from build123d import *

# Parameters (mm, degrees)
CUT_EXTRUDE_1_DEPTH = 3
FILLET_1_R          = 1
CHAMFER_1_SIZE      = 0.5


with BuildPart() as part:
    # 草图1 → 旋转1 (revolve)
    with BuildSketch(Plane.XY):
        Polygon((0, 0), (0, 5), (4.5, 5), (4.5, 3), (20.5, 3), (20.5, 2.5), (30.5, 2.5), (30.5, 0), align=None)
    revolve(axis=Axis((0, 0, 0), (1, 0, 0)))

    # 草图2 → 切除-拉伸1 (cut)
    with BuildSketch(Plane.ZY):
        Polygon((0, 1.732050808), (-1.5, 0.866025404), (-1.5, -0.866025404), (0, -1.732050808), (1.5, -0.866025404), (1.5, 0.866025404), align=None)
    extrude(amount=-CUT_EXTRUDE_1_DEPTH, mode=Mode.SUBTRACT)

    # 圆角1
    fillet_1_edges = [part.edges().sort_by_distance(p)[0] for p in [
        (0, -5, 0),
    ]]
    fillet(fillet_1_edges, radius=FILLET_1_R)

    # 倒角1
    chamfer_1_edges = [part.edges().sort_by_distance(p)[0] for p in [
        (30.5, -2.5, 0),
    ]]
    chamfer(chamfer_1_edges, length=CHAMFER_1_SIZE)


solid = part.part
CAD build for the part. Positions are in the model's coordinates, mm. A direction names the side the tool comes from. Give positions to 0.01 mm unless a question says otherwise; leave off trailing zeros. Loops run counter-clockwise (first coordinate to the right, second up) from the corner with the lowest first, then second, coordinate; pieces in that order, holes last. Notation, with made-up numbers: M -32,33.25 L 10,33.25 A7 ccw 10,44.25 Z; hole C 80.25,17.5 d1. An arc over 180 degrees is marked long. Answer in a Markdown table with one row per item. Add a question column.
Item 1: Tool access for faces 1 (the face through (13, -3, 0)), 2 (the face through (0, -2, 0)), 3 (the face through (3, 0, 0)): list every direction of +Z, -Z, +X, -X, +Y, -Y with a clear straight run to the whole face (end or side of a thin tool).
Item 2: Band-saw the part on C-C on x = 22. Give the cut face in (y, z).
Item 3: Probe probe 1 along Z at (x, y) = (29, -2); probe 2 along X at (y, z) = (-1.5, -2.5); probe 3 along X at (y, z) = (-3.5, -0.25). List the from-to ranges inside material, lowest first.
Item 4: Band-saw the part on B-B on x = 8. Give the cut face in (y, z), then the cut area to 3 significant figures.
Item 5: Band-saw the part on A-A on y = 0. Give the cut face in (x, z), then the cut area to 3 significant figures.
Item 6: Drop flat-ended pins along their axis: P1, Ø3, axis at y = 2.5, z = 0, coming from the -X side; P2, Ø0.5, axis at x = 2, y = 0.5, coming from the -Z side; P3, Ø4, axis at x = 21, y = -2, coming from the -Z side; P4, Ø2, axis at x = 23, z = -1.5, coming from the -Y side. Give the stop position or say it passes through.
Item 7: Mould opens along Z. For faces 4 (the face through (30.5, 0, 0)), 5 (the face through (1.479, -1.293, -0.76)), 6 (the face through (2.77, -1.08, -4.88)) say: +Z half, -Z half, draft (parallel to the pull), parting line (faces both ways), or undercut.
Reply:
| question | item | result |
|---|---|---|
| 1 | face 1 | +X |
| 1 | face 2 | +Z, -Z, -X, +Y, -Y |
| 1 | face 3 | -X |
| 2 | outline | C 0,0 d5 |
| 3 | probe 1 | z = -1.5 to 1.5 |
| 3 | probe 2 | x = 0 to 20.5 |
| 3 | probe 3 | x = 0 to 4.5 |
| 4 | outline | C 0,0 d6 |
| 4 | area | 28.3 mm^2 |
| 5 | outline | M 0,-4 A1 ccw 1,-5 L 4.5,-5 L 4.5,-3 L 20.5,-3 L 20.5,-2.5 L 30,-2.5 L 30.5,-2 L 30.5,2 L 30,2.5 L 20.5,2.5 L 20.5,3 L 4.5,3 L 4.5,5 L 1,5 A1 ccw 0,4 L 0,1.5 L 3,1.5 L 3,-1.5 L 0,-1.5 Z |
| 5 | area | 181 mm^2 |
| 6 | P1 | stops at x = 0 |
| 6 | P2 | stops at z = -4.99 |
| 6 | P3 | stops at z = -3 |
| 6 | P4 | stops at y = -2.45 |
| 7 | face 4 | draft |
| 7 | face 5 | undercut |
| 7 | face 6 | parting line |
